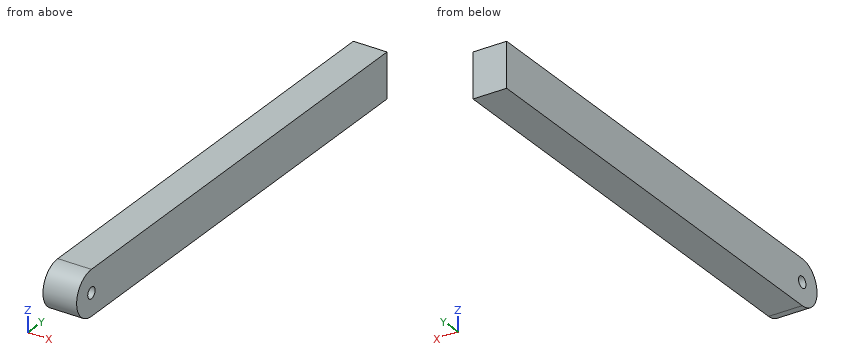
from build123d import *

# Parameters (mm, degrees)
ESQUISSE3_R = 2.5
BASE_DEPTH  = 15


with BuildPart() as part:
    # Esquisse3 → BASE (new body)
    with BuildSketch(Plane(origin=(0, 0, 0), x_dir=(0, 0, -1), z_dir=(1, 0, 0))):
        with BuildLine():
            Line((10, 100), (-10, 100))
            Line((-10, 100), (-10, -100))
            ThreePointArc((-10, -100), (0, -110), (10, -100))
            Line((10, -100), (10, 100))
        make_face()
        with Locations((0, -100)):
            Circle(ESQUISSE3_R, mode=Mode.SUBTRACT)
    extrude(amount=BASE_DEPTH)


solid = part.part
Input: part model. Units: mm. Frame: model coordinates. Coordinates: 2 decimals unless noted, no trailing zeros. Write each loop counter-clockwise with the first axis right and the second up, starting at its lowest first coordinate (ties: lowest second). Pieces come first, ordered by that corner, then holes. Notation, with made-up numbers: M -20.5,45 L 14.5,45 A25 ccw 14.5,78 Z; hole C 47.5,65.25 d1. An arc over 180 degrees is marked long. Answer as a JSON object with one key per item and string values. Group by question number.
(1) Section A-A on z = 0. Output: boundary loops of the cut face in (x, y), plus the area to 4 significant figures.
(2) Ray query, line 1 along Y through (x, z) = (7.25, 0); line 2 along Y through (x, z) = (2.5, -0.5); line 3 along Y through (x, z) = (12, -6.5). Return the intervals inside material, ascending. Write a range as [from, to].
(3) Section B-B on z = 7.5. Output: boundary loops of the cut face in (x, y), plus the area to 3 significant figures.
(4) Contact query for a flat-ended pin moving along its axis: P1, Ø3, axis at x = 11, z = 7, coming from the -Y side. Output: stop coordinate, or through.
Result set:
{
 "1": {"outline": "M 0,-110 L 15,-110 L 15,-102.5 L 0,-102.5 Z; M 0,-97.5 L 15,-97.5 L 15,100 L 0,100 Z", "area": "3,075 mm2"},
 "2": {"line 1": "y = [-110, -102.5], [-97.5, 100]", "line 2": "y = [-109.99, -102.45], [-97.55, 100]", "line 3": "y = [-107.6, 100]"},
 "3": {"outline": "M 0,-106.61 L 15,-106.61 L 15,100 L 0,100 Z", "area": "3,100 mm2"},
 "4": {"P1": "stops at y = -108.35"}
}
